```python
from build123d import *

# Parameters (mm, degrees)
SKETCH2_R           = 2.38125
SKETCH2_R_2         = 1.85
BOSS_EXTRUDE1_DEPTH = 4.318


with BuildPart() as part:
    # Sketch2 → Boss-Extrude1 (new body)
    with BuildSketch(Plane(origin=(0, 0, 0), x_dir=(0, 0, -1), z_dir=(1, 0, 0))):
        with BuildLine():
            Line((-115.889220019, 171.954), (-219.799081889, 171.954))
            ThreePointArc((-219.799081889, 171.954), (-224.603807745, 170.72409746), (-228.226664693, 167.336921891))
            Line((-228.226664693, 167.336921891), (-294.933682845, 62.899419265))
            ThreePointArc((-294.933682845, 62.899419265), (-295.905218473, 53.919072951), (-289.341021135, 47.714089896))
            Line((-289.341021135, 47.714089896), (-238.759677477, 32.254))
            Line((-238.759677477, 32.254), (-202.359677477, -1.524))
            Line((-202.359677477, -1.524), (-189.18491037, -1.524))
            Line((-189.18491037, -1.524), (-183.068077693, 7.544577378))
            Line((-183.068077693, 7.544577378), (-179.720203102, 5.286407453))
            Line((-179.720203102, 5.286407453), (-184.313880932, -1.524))
            Line((-184.313880932, -1.524), (-158.188157254, -1.524))
            ThreePointArc((-158.188157254, -1.524), (-147.265506636, 25.180552261), (-120.759258716, 36.576))
            Line((-120.759258716, 36.576), (-120.759258716, 66.032))
            Line((-120.759258716, 66.032), (-105.889220019, 88.077738973))
            Line((-105.889220019, 88.077738973), (-105.889220019, 161.954))
            ThreePointArc((-105.889220019, 161.954), (-108.818152207, 169.025067812), (-115.889220019, 171.954))
        make_face()
        with Locations((-286.371258716, 57.430370624)):
            Circle(SKETCH2_R, mode=Mode.SUBTRACT)
        with Locations((-229.557259723, 141.660587995)):
            Circle(SKETCH2_R, mode=Mode.SUBTRACT)
        with Locations((-112.732319414, 86.216867448)):
            Circle(SKETCH2_R_2, mode=Mode.SUBTRACT)
        with Locations((-199.955990958, 72)):
            Circle(SKETCH2_R_2, mode=Mode.SUBTRACT)
        with Locations((-199.955990958, 152)):
            Circle(SKETCH2_R_2, mode=Mode.SUBTRACT)
        with Locations((-199.955990958, 168)):
            Circle(SKETCH2_R_2, mode=Mode.SUBTRACT)
        with Locations((-199.955990958, 40)):
            Circle(SKETCH2_R_2, mode=Mode.SUBTRACT)
        with Locations((-191.955990958, 48)):
            Circle(SKETCH2_R_2, mode=Mode.SUBTRACT)
        with Locations((-199.955990958, 56)):
            Circle(SKETCH2_R_2, mode=Mode.SUBTRACT)
    extrude(amount=BOSS_EXTRUDE1_DEPTH)


solid = part.part
```
Work out the finished part from the listing and answer in its coordinate system (mm). A direction names the side the tool comes from. Coordinates: 2 decimals unless noted, no trailing zeros. Write each loop counter-clockwise with the first axis right and the second up, starting at its lowest first coordinate (ties: lowest second). Pieces come first, ordered by that corner, then holes. Notation, with made-up numbers: (-5.75, -34.5) - (6.25, -34.5) arc R7 cw to (6.25, -22.5) - close; hole circle Ø3 at (-4, 35). An arc over 180 degrees is marked (long way). Answer as a JSON object with one key per item and string values.
Q1. Find section B-B (y = 159). Write down the section's boundary in (x, z), plus the area to 3 significant figures.
Results list:
{"outline": "(0, 105.89) - (4.32, 105.89) - (4.32, 233.55) - (0, 233.55) - close", "area": "551 mm^2"}
Q2. Consider L1, parallel to Z at x = 0.85, y = 57; L2, parallel to Z at x = 3.35, y = 152; L3, parallel to Z at x = 3.4, y = 25. Determine where each line is inside the solid, lowest interval first. Write a range as from..to.
Results list:
{"L1": "z = 120.76..198.4, 201.51..284.03, 288.71..296.52", "L2": "z = 105.89..198.11, 201.81..238.02", "L3": "z = 147.44..230.94"}
Q3. Find section C-C (z = 139). Write down the section's boundary in (x, y), plus the area to 3 significant figures.
Results list:
{"outline": "(0, 31.55) - (4.32, 31.55) - (4.32, 171.95) - (0, 171.95) - close", "area": "606 mm^2"}
Q4. Find section A-A (x = 2.95). State how many separate pieces and enclosed holes the cut face has, plus the area to 3 significant figures.
Results list:
{"separate pieces": "1", "enclosed holes": "9", "area": "23,600 mm^2"}
Q5. For a pull along Y with two mould halves and no side action, classify faces 1 (the cylindrical face through (2.13, 54.04, 295.95)), 2 (the flat face through (2.129, 115.849, 261.113)), 3 (the flat face through (2.1, 2.9, 186.2)), 4 (the flat face through (2, 51, 120.759)) as pulls with the +Y half, pulls with the -Y half, needs draft (parallel to the pull), parting line crosses it, or undercut.
Results list:
{"face 1": "parting line crosses it", "face 2": "pulls with the +Y half", "face 3": "undercut", "face 4": "needs draft"}
Q6. Which of the six approach directions +Z, -Z, +X, -X, +Y, -Y give full straight-line access (tool end or side, diameter ignored) to faces 5 (the flat face through (2.129, 1.929, 181.985)), 6 (the flat face through (2.13, 40.09, 264.4))?
Results list:
{"face 5": "+X, -X", "face 6": "+Z, +X, -X, -Y"}
